Drawing for the job (mm, zero at the part's lowest x, y, z). Round coordinates to 2 decimals unless told otherwise and drop trailing zeros. Loops run counter-clockwise (first coordinate to the right, second up) from the corner with the lowest first, then second, coordinate; pieces in that order, holes last. Notation, with made-up numbers: M 23,84 L 65,84 A15 ccw 65,88 Z; hole C 18,-32.5 d3. An arc over 180 degrees is marked long. Use a Markdown table: item, result. Add a question column.
Q1. Cut at A-A (z = 1.75). Give the cut face in (x, y), plus the area to 3 significant figures.
Q2. Probe line 1 (X direction, y = 3, z = 2.55); line 2 (Y direction, x = 1.75, z = 2.05); line 3 (X direction, y = 5, z = 2.15). List the from-to ranges inside material, lowest first. Write a range as from..to.
Q3. Cut at B-B (y = 3). Give the cut face in (x, z), plus the area to 3 significant figures.
Q4. Cut at C-C (x = 4). Give the cut face in (y, z).
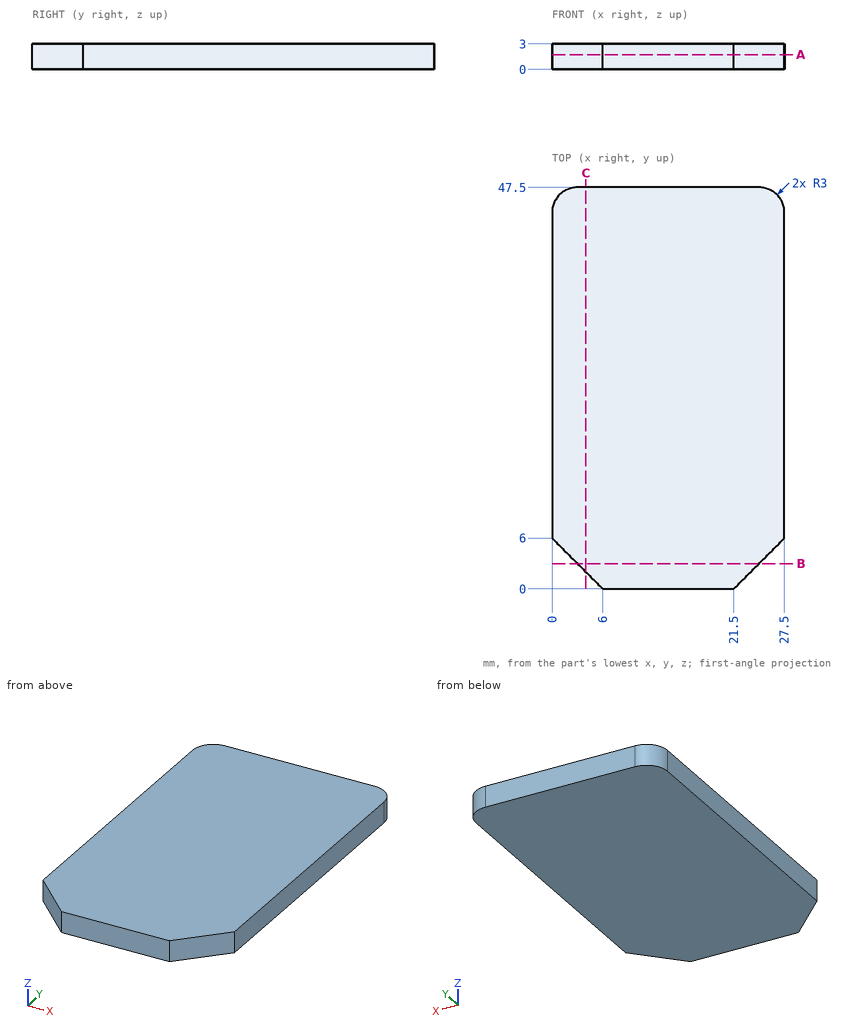
Checked values:
| question | item | result |
|---|---|---|
| 1 | outline | M 0,6 L 6,0 L 21.5,0 L 27.5,6 L 27.5,44.5 A3 ccw 24.5,47.5 L 3,47.5 A3 ccw 0,44.5 Z |
| 1 | area | 1,270 mm^2 |
| 2 | line 1 | x = 3..24.5 |
| 2 | line 2 | y = 4.25..47.23 |
| 2 | line 3 | x = 1..26.5 |
| 3 | outline | M 3,0 L 24.5,0 L 24.5,3 L 3,3 Z |
| 3 | area | 64.5 mm^2 |
| 4 | outline | M 2,0 L 47.5,0 L 47.5,3 L 2,3 Z |
